Can you work these out from the model? Positions are in its coordinate system, mm. Face numbers are marked on the shaded views. A direction names the side the tool comes from. Round coordinates to 2 decimals unless told otherwise and drop trailing zeros. Loops run counter-clockwise (first coordinate to the right, second up) from the corner with the lowest first, then second, coordinate; pieces in that order, holes last.
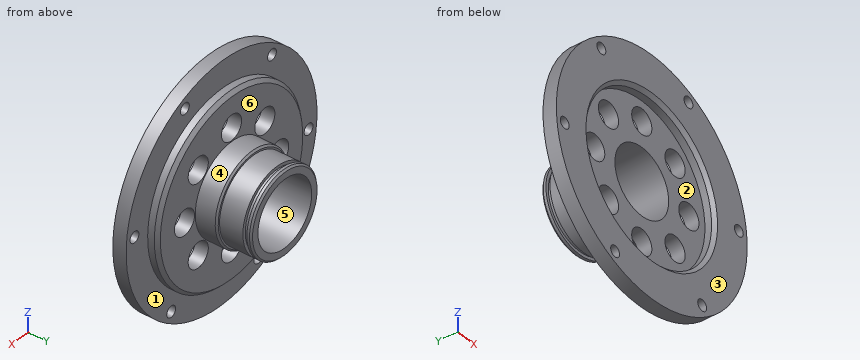
from build123d import *

# Parameters (mm, degrees)
SKETCH_2_R               = 3.75
CUT_EXTRUDE_1_DEPTH      = 10
CHAMFER_1_SIZE           = 1
CHAMFER_2_SIZE           = 1
SKETCH_3_W               = 0.9
SKETCH_3_H               = 1.2
CHAMFER_3_SIZE           = 0.5
HOLE_WIZARD_M4_1_D       = 3.3
PATTERN_CIRCULAR_1_COUNT = 6
SKETCH_7_R               = 13.5
SKETCH_7_R_2             = 12.5
EXTRUDE_1_DEPTH          = 6.5
CHAMFER_4_SIZE           = 0.5


with BuildPart() as part:
    # 草图1 → 旋转1 (revolve)
    with BuildSketch(Plane.XY, mode=Mode.PRIVATE) as revolve_1_sk:
        Polygon((-35.475, 0), (-23.475, 0), (-23.475, 3), (-10, 3), (-10, 23), (-12.5, 23), (-12.5, 7), (-27.475, 7), (-27.475, 4), (-35.475, 4), align=None)
    revolve(revolve_1_sk.sketch.rotate(Axis((0, 0, 0), (0, 1, 0)), 270), axis=Axis((0, 0, 0), (0, 1, 0)))

    # 草图2 → 切除-拉伸1 (cut)
    with BuildSketch(Plane(origin=(0, 7, 0), x_dir=(1, 0, 0), z_dir=(0, 1, 0))):
        with Locations(Location((0, 17.5, 0), (0, 0, 270))):
            Circle(SKETCH_2_R)
        with Locations(Location((12.374368671, 12.374368671, 0), (0, 0, 270))):
            Circle(SKETCH_2_R)
        with Locations(Location((17.5, 0, 0), (0, 0, 270))):
            Circle(SKETCH_2_R)
        with Locations(Location((12.374368671, -12.374368671, 0), (0, 0, 270))):
            Circle(SKETCH_2_R)
        with Locations(Location((0, -17.5, 0), (0, 0, 270))):
            Circle(SKETCH_2_R)
        with Locations(Location((-12.374368671, -12.374368671, 0), (0, 0, 270))):
            Circle(SKETCH_2_R)
        with Locations(Location((-17.5, 0, 0), (0, 0, 270))):
            Circle(SKETCH_2_R)
        with Locations(Location((-12.374368671, 12.374368671, 0), (0, 0, 270))):
            Circle(SKETCH_2_R)
    extrude(amount=-CUT_EXTRUDE_1_DEPTH, mode=Mode.SUBTRACT)

    # 倒角1
    chamfer_1_edges = [part.edges().sort_by_distance(p)[0] for p in [
        (0, 0, 23.475),
    ]]
    chamfer(chamfer_1_edges, length=CHAMFER_1_SIZE)

    # 倒角2
    chamfer_2_edges = [part.edges().sort_by_distance(p)[0] for p in [
        (0, 7, 27.475),
    ]]
    chamfer(chamfer_2_edges, length=CHAMFER_2_SIZE)

    # 草图3 → 切除-旋转1 (revolve, cut)
    with BuildSketch(Plane.XY, mode=Mode.PRIVATE) as cut_revolve_1_sk:
        with Locations((12.05, 21.1)):
            Rectangle(SKETCH_3_W, SKETCH_3_H)
    revolve(cut_revolve_1_sk.sketch.rotate(Axis((0, 0, 0), (0, 1, 0)), 90), axis=Axis((0, 0, 0), (0, 1, 0)), mode=Mode.SUBTRACT)

    # 倒角3
    chamfer_3_edges = [part.edges().sort_by_distance(p)[0] for p in [
        (0, 23, 12.5),
    ]]
    chamfer(chamfer_3_edges, length=CHAMFER_3_SIZE)

    # M4 螺纹孔1 (through all)
    with Locations(Plane(origin=(0, 4, 0), x_dir=(1, 0, 0), z_dir=(0, 1, 0))):
        with Locations((18.734776664, 26.55669677)):
            hole_wizard_m4_1 = Hole(HOLE_WIZARD_M4_1_D / 2)

    # 阵列(圆周)1: M4 螺纹孔1 ×6 about axis
    pattern_circular_1_axis = Axis((0, 0, 0), (0, 1, 0))
    for i in range(1, PATTERN_CIRCULAR_1_COUNT):
        add(hole_wizard_m4_1.rotate(pattern_circular_1_axis, i * 360 / PATTERN_CIRCULAR_1_COUNT), mode=Mode.SUBTRACT)

    # 草图7 → 凸台-拉伸1 (add)
    with BuildSketch(Plane(origin=(0, 7, 0), x_dir=(1, 0, 0), z_dir=(0, 1, 0))):
        with Locations(Location((0, 0, 0), (0, 0, 90))):
            Circle(SKETCH_7_R)
        with Locations(Location((0, 0, 0), (0, 0, 90))):
            Circle(SKETCH_7_R_2, mode=Mode.SUBTRACT)
    extrude(amount=EXTRUDE_1_DEPTH)

    # 倒角4
    chamfer_4_edges = [part.edges().sort_by_distance(p)[0] for p in [
        (0, 13.5, 13.5),
    ]]
    chamfer(chamfer_4_edges, length=CHAMFER_4_SIZE)


solid = part.part
(1) If we section it at A-A, the plane z = 0: State how many separate pieces and enclosed holes the cut face has, then the cut area to 3 significant figures.
Worked answers:
separate pieces: 4
enclosed holes: 0
area: 256 mm2
(2) Will these pins go through, and if not, where does the flat tip stop? P1, Ø4, axis at y = 17, z = -8.5, coming from the +X side; P2, Ø10, axis at y = 17.5, z = 12.5, coming from the +X side; P3, Ø10, axis at y = 16.5, z = 8.5, coming from the -X side.
Worked answers:
P1: stops at x = 10.68
P2: stops at x = 10
P3: stops at x = -12.57
(3) If we section it at C-C, the plane y = 12: List the corners of the cut face in (x, z) for me, then the cut area to 3 significant figures.
Worked answers:
outline: circle Ø27 at (0, 0); hole circle Ø20 at (0, 0)
area: 258 mm2
(4) For the marked faces 1, 2 and 3, which set-ups out of +Z, -Z, +X, -X, +Y, -Y let a thin tool reach every point of the face, with its end or its side?
Worked answers:
face 1: +Y
face 2: -Y
face 3: +Z, -Z, +X, -X, -Y
(5) If we mould it in two halves opening along Z, with no side actions, what happens to the marked faces 4, 5 and 6? For each: released by +Z, released by -Z, zero draft, split by the parting line, or undercut.
Worked answers:
face 4: split by the parting line
face 5: undercut
face 6: zero draft
(6) If I drill on line 1 (X direction, y = 1.25, z = 10); line 2 (Y direction, x = 22, z = -11); line 3 (Y direction, x = 30, z = 10.5), over which ranges is the centre line in solid material (lowest first)?
Worked answers:
line 1: x = -34.04 to -21.24, 21.24 to 34.04
line 2: y = 0 to 7
line 3: y = 0 to 4
